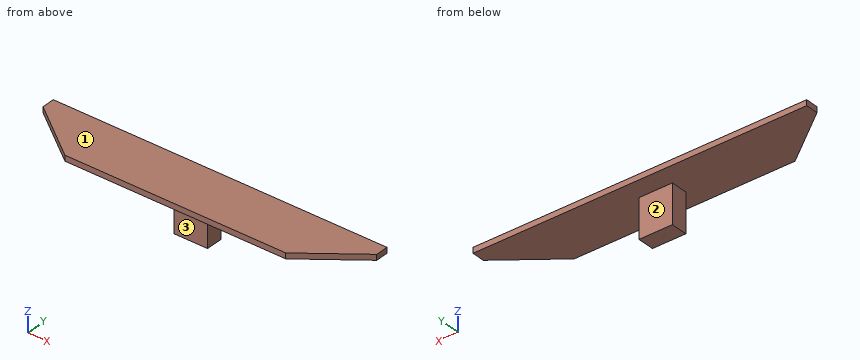
from build123d import *

# Parameters (mm, degrees)
F0_W     = 7.62
F0_H     = 17.78
F1_DEPTH = 7.62
F2_W     = 25.4
F2_H     = 2.54
F3_DEPTH = 76.2
F5_DEPTH = 50.8


with BuildPart() as f1:
    # F0 (on Right) → F1 (new body)
    with BuildSketch(Plane.YZ):
        with Locations((18.735414, -6.280092)):
            Rectangle(F0_W, F0_H)
    extrude(amount=F1_DEPTH)

    # F2 (on Right) → F3 (join)
    with BuildSketch(Plane.YZ):
        with Locations((18.816974, 3.868257)):
            Rectangle(F2_W, F2_H)
    extrude(amount=F3_DEPTH)

    # F4 (on face) → F5 (cut)
    with BuildSketch(Plane.XY.offset(5.138257)):
        Polygon((76.2, 6.116974), (76.2, 25.691286), (50.403856, 6.116974), align=None)
    extrude(amount=-F5_DEPTH, mode=Mode.SUBTRACT)

    # F6: F1 across plane


with BuildPart() as f1_1:
    add(f1.part)
    add(f1.part.mirror(Plane.YZ))


solid = f1_1.part
Could you check a few things on this model? Use its own coordinates, in mm. Face numbers are marked on the shaded views. A direction names the side the tool comes from. Coordinates: 2 decimals unless noted, no trailing zeros. Order: outer loops, then holes, each group sorted by start corner. A loop starts at its lowest first (then second) coordinate and runs counter-clockwise, first axis right, second up. Notation, with made-up numbers: (53, 85.25) -> (86, 85.25) arc R17 ccw to (86, 96.25) -> close; hole circle Ø2 at (1, 51). An arc over 180 degrees is marked (long way). One line per item, written item: value. Start each with the question number.
1) Imagine slicing it at A-A on y = 16.25. List the corners of the cut face in (x, z) for me.
2) Imagine slicing it at B-B on z = 0.25. List the corners of the cut face in (x, y) for me, plus the area to 3 significant figures.
3) I'm going to push flat-ended pins straight in: pin 1 (4.5 mm diameter, centred on x = 1.5, z = -2, fed in from -Y); pin 2 (2.5 mm diameter, centred on y = 20, z = -8, fed in from -X); pin 3 (1.5 mm diameter, centred on x = -24, y = 17, fed in from -Z); pin 4 (10 mm diameter, centred on x = -18.5, z = 1.5, fed in from +Y). Where does each tip first touch, or does it pass through?
4) If I drill on L1, parallel to Z at x = 23.5, y = 20; L2, parallel to X at y = 18.75, z = -7; L3, parallel to Y at x = 7.5, z = -2, over which ranges is the centre line in solid material (lowest first)? Write a range as [from, to].
5) Imagine slicing it at C-C on x = 35. List the corners of the cut face in (y, z) for me.
6) Which directions (+Z, -Z, +X, -X, +Y, -Y) give clear straight access to the entire face, cutting with the end or side of a thin tool? Please do the marked faces 1, 2 and 3.
Answer list:
1. outline: (-63.76, 2.6) -> (-7.62, 2.6) -> (-7.62, -15.17) -> (7.62, -15.17) -> (7.62, 2.6) -> (63.76, 2.6) -> (63.76, 5.14) -> (-63.76, 5.14) -> close
2. outline: (-7.62, 14.93) -> (7.62, 14.93) -> (7.62, 22.55) -> (-7.62, 22.55) -> close
2. area: 116 mm2
3. pin 1: stops at y = 14.93
3. pin 2: stops at x = -7.62
3. pin 3: stops at z = 2.6
3. pin 4: stops at y = 31.52
4. L1: z = [2.6, 5.14]
4. L2: x = [-7.62, 7.62]
4. L3: y = [14.93, 22.55]
5. outline: (6.12, 2.6) -> (31.52, 2.6) -> (31.52, 5.14) -> (6.12, 5.14) -> close
6. face 1: +Z, +X, -X, +Y, -Y
6. face 2: -Z, +X, -X, +Y
6. face 3: -Z, +X, -X, -Y
